Source: CAD feature listing. Evaluate the final solid. Frame: model axes, mm. Face numbers are marked on the shaded views. A direction names the side the tool comes from. Coordinates: 2 decimals unless noted, no trailing zeros. Write each loop counter-clockwise with the first axis right and the second up, starting at its lowest first coordinate (ties: lowest second). Pieces come first, ordered by that corner, then holes. Notation, with made-up numbers: M 0,-3 L 50,-3 A14 cw 50,15 Z; hole C 46.25,-3 d3. An arc over 180 degrees is marked long. One line per item, written item: value. Start each with the question number.
Item 1: Ray query, L1, parallel to Y at x = -3.6, z = 0; L2, parallel to X at y = 2.5, z = 0.5; L3, parallel to Y at x = 3.25, z = -1.5. Return the intervals inside material, ascending. Write a range as from..to.
Item 2: Set-up query: the marked faces 1 and 2. Return all of +Z, -Z, +X, -X, +Y, -Y with unobstructed straight access to the full face (end or side cutting, diameter ignored); none if empty.
Item 3: Cut plane B-B, the plane y = 5. Output: boundary loops of the cut face in (x, z), then the cut area to 3 significant figures.
Item 4: Cut plane C-C, the plane x = 0.75. Output: boundary loops of the cut face in (y, z), then the cut area to 3 significant figures.
Item 5: Mould query, pull axis Y, two halves, no side actions, for the marked faces 3, 4 and 5. Classes: released by +Y, released by -Y, zero draft, split by the parting line, or undercut.
Item 6: Cut plane A-A, the plane z = 0. Output: boundary loops of the cut face in (x, y), then the cut area to 3 significant figures.
Item 7: Pin query (flat end, axial travel): P1, Ø3.5, axis at y = 3.5, z = -0.5, coming from the +X side; P2, Ø1.5, axis at x = 1, z = 2, coming from the +Y side. Return the tip coordinate at first contact, or that it passes through.
Item 8: Cut plane D-D, the plane y = 6. Output: boundary loops of the cut face in (x, z), then the cut area to 3 significant figures.
Autodesk Inventor part; units mm, degrees
ref_plane "YZ Plane" through (0, 0, 0) normal (1, 0, 0) x (0, 1, 0)
ref_plane "XZ Plane" through (0, 0, 0) normal (0, 1, 0) x (-1, 0, 0)
ref_plane "XY Plane" through (0, 0, 0) normal (0, 0, 1) x (1, 0, 0)
sketch "Sketch1" plane through (0, 0, 0) normal (0, 1, 0) x (-1, 0, 0)
  line L0 (5, 5) -> (-5, 5)
  line L1 (-5, 5) -> (-5, -5)
  line L2 (-5, -5) -> (5, -5)
  line L3 (5, -5) -> (5, 5)
  line L4 (5, 5) -> (-5, -5) construction
  line L5 (-5, 5) -> (5, -5) construction
  point P0 (0, 0)
  dimension "d0" = 10
  dimension "d1" = 10
extrude "Extrusion1" add sketch "Sketch1" along normal blind 1.5
sketch "Sketch2" plane through (0, 1.5, 0) normal (0, 1, 0) x (1, 0, 0)
  line L0 (-5, -5) -> (5, -5)
  line L1 (5, 5) -> (-5, 5)
  line L2 (-5, -5) -> (-3, -5)
  line L3 (-3, -5) -> (-3, 5)
  line L4 (-3, 5) -> (-5, 5)
  line L5 (-5, 5) -> (-5, -5)
  point P0 (0, 0)
  dimension "d4" = 2
extrude "Extrusion2" add sketch "Sketch2" along normal blind 7
sketch "Sketch3" plane through (-5, 0, -5) normal (-1, 0, 0) x (0, 0, 1)
  circle A0 centre (5, 5) radius 2.25
  line L0 (0, 0) -> (10, 0)
  line L1 (0, 0) -> (0, 8.5)
  point P0 (5, 0)
  dimension "d7" = 4.5
  dimension "d8" = 5
  dimension "d9" = 5
extrude "Extrusion3" cut sketch "Sketch3" against normal through all
fillet "Fillet1" radius 2 2 edges at (-4, 8.5, 5) (-4, 8.5, -5)
properties part number "screw_holder"
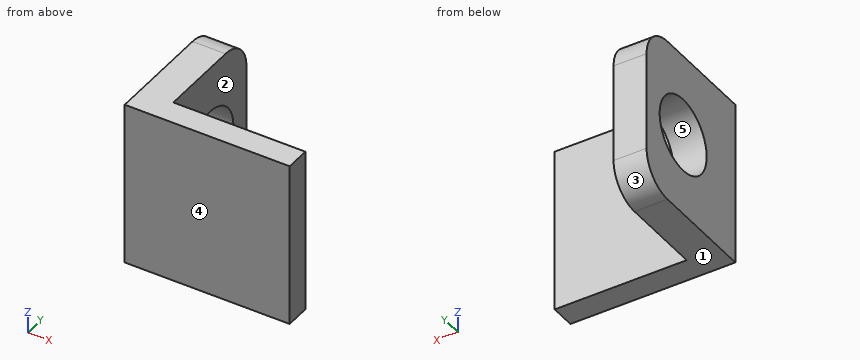
From the geometry:
1. L1: y = 0..2.75, 7.25..8.5
1. L2: x = -5..-3
1. L3: y = 0..1.5
2. face 1: -Z, +X, -X, +Y, -Y
2. face 2: +Z, -Z, +X, +Y
3. outline: M -5,-5 L -3,-5 L -3,-2.25 L -5,-2.25 Z; M -5,2.25 L -3,2.25 L -3,5 L -5,5 Z
3. area: 11.0 mm²
4. outline: M 0,-5 L 1.5,-5 L 1.5,5 L 0,5 Z
4. area: 15.0 mm²
5. face 3: released by +Y
5. face 4: released by -Y
5. face 5: undercut
6. outline: M -5,0 L 5,0 L 5,1.5 L -3,1.5 L -3,2.75 L -5,2.75 Z; M -5,7.25 L -3,7.25 L -3,8.5 L -5,8.5 Z
6. area: 20.0 mm²
7. P1: stops at x = -3
7. P2: stops at y = 1.5
8. outline: M -5,-5 L -3,-5 L -3,-2.02 L -5,-2.02 Z; M -5,2.02 L -3,2.02 L -3,5 L -5,5 Z
8. area: 11.9 mm²
